The model under review builds one solid part; all positions refer to its coordinate system, in mm. A direction names the side the tool comes from. Give positions to 0.01 mm unless a question says otherwise; leave off trailing zeros. Order: outer loops, then holes, each group sorted by start corner. A loop starts at its lowest first (then second) coordinate and runs counter-clockwise, first axis right, second up. Notation, with made-up numbers: (39, -18) - (73, -18) arc R12 ccw to (73, -6) - close; hole circle Ø6 at (45, 16). An arc over 180 degrees is marked (long way). Use CSV: the item, a comma, the result in double quotes. Start each with the question number.
1. Machinability: for faces 1 (the flat face through (5, 2, -22)), 2 (the flat face through (-22, 2, -5)), 3 (the flat face through (7.42, 3.1, 2.57)), which of the approach directions +Z, -Z, +X, -X, +Y, -Y give a long, thin tool a straight path to every point of the face, cutting with its end or side? Answer none if there is none.
2. To check wall thickness, follow line 1 (Z direction, x = -1, y = 2.9); line 2 (Z direction, x = -27.5, y = 2.85); line 3 (X direction, y = 0.85, z = -22). State the ranges of each line that lie inside material, in increasing order. Write a range as [from, to].
3. Take a section at A-A, the plane x = -24. State the section outline as (y, z) points, then the cut area to 3 significant figures.
4. Draft analysis for pull direction X (two halves, no side actions). For faces 4 (the cylindrical face through (-32.7, 1.7, -0.1)), 5 (the conical face through (-0.817, 0.484, 16.921)), 6 (the flat face through (5, 2, 22)), state which applies: released by +X, released by -X, zero draft, split by the parting line, or undercut.
5. Take a section at B-B, the plane y = 0.85. Count the separate pieces of the cut face and the enclosed holes in it, then the cut area to 3 significant figures.
6. For pin 1 (0.9 mm diameter, centred on x = 22.5, y = 1, fed in from +Z); pin 2 (1.5 mm diameter, centred on x = 12, y = 1, fed in from +Z); pin 3 (0.9 mm diameter, centred on x = 20.5, y = 1.5, fed in from -Z), all flat-tipped, find the tip position at first contact; note any pin that passes through.
```python
from build123d import *

# Parameters (mm, degrees)
SKETCH1_R           = 7.45
SKETCH1_R_2         = 2
BOSS_EXTRUDE1_DEPTH = 3.1
CIRPATTERN1_COUNT   = 4
CHAMFER3_SIZE       = 0.25
CHAMFER4_SIZE       = 2.75
CHAMFER5_SIZE       = 0.25


with BuildPart() as part:
    # Sketch1 → Boss-Extrude1 (new body)
    with BuildSketch(Plane(origin=(0, 0, 0), x_dir=(1, 0, 0), z_dir=(0, 1, 0))):
        with BuildLine():
            Line((5, 16.58427681), (5, 27.7))
            ThreePointArc((5, 27.7), (0, 32.7), (-5, 27.7))
            Line((-5, 27.7), (-5, 16.58427681))
            ThreePointArc((-5, 16.58427681), (-4.969037433, 15.767138405), (-5, 14.95))
            ThreePointArc((-5, 14.95), (-5.95461278, 11.260107735), (-8.131727984, 8.131727984))
            ThreePointArc((-8.131727984, 8.131727984), (0, -11.5), (8.131727984, 8.131727984))
            ThreePointArc((8.131727984, 8.131727984), (5.95461278, 11.260107735), (5, 14.95))
            ThreePointArc((5, 14.95), (4.969037433, 15.767138405), (5, 16.58427681))
        make_face()
        with Locations(Location((0, 0, 0), (0, 0, 90))):
            Circle(SKETCH1_R, mode=Mode.SUBTRACT)
        with Locations(Location((0, 14.95, 0), (0, 0, 90))):
            Circle(SKETCH1_R_2, mode=Mode.SUBTRACT)
        with Locations(Location((0, 27.7, 0), (0, 0, 90))):
            Circle(SKETCH1_R_2, mode=Mode.SUBTRACT)
    extrude(amount=BOSS_EXTRUDE1_DEPTH)


with BuildPart() as cirpattern1_1:
    # CirPattern1: pattern copy
    add(part.part.rotate(Axis((0, 0, 0), (0, 1, 0)), 1 * 360 / CIRPATTERN1_COUNT))


with BuildPart() as cirpattern1_2:
    # CirPattern1: pattern copy
    add(part.part.rotate(Axis((0, 0, 0), (0, 1, 0)), 2 * 360 / CIRPATTERN1_COUNT))


with BuildPart() as cirpattern1_3:
    # CirPattern1: pattern copy
    add(part.part.rotate(Axis((0, 0, 0), (0, 1, 0)), 3 * 360 / CIRPATTERN1_COUNT))


with BuildPart() as cirpattern1_1_1:
    add(cirpattern1_1.part)

    # Combine1: union part, CirPattern1_3, CirPattern1_2
    add(part.part)
    add(cirpattern1_3.part)
    add(cirpattern1_2.part)

    # Chamfer3
    chamfer3_edges = [cirpattern1_1_1.edges().sort_by_distance(p)[0] for p in [
        (-25.7, 3.1, 0),
        (0, 3.1, -25.7),
        (25.7, 3.1, 0),
        (0, 3.1, 25.7),
        (7.45, 3.1, 0),
    ]]
    chamfer(chamfer3_edges, length=CHAMFER3_SIZE)

    # Chamfer4
    chamfer4_edges = [cirpattern1_1_1.edges().sort_by_distance(p)[0] for p in [
        (-12.95, 3.1, 0),
        (0, 3.1, -12.95),
        (12.95, 3.1, 0),
        (0, 3.1, 12.95),
    ]]
    chamfer(chamfer4_edges, length=CHAMFER4_SIZE)

    # Chamfer5
    chamfer5_edges = [cirpattern1_1_1.edges().sort_by_distance(p)[0] for p in [
        (-32.7, 0, 0),
        (-22.142138405, 0, -5),
        (-8.131727984, 0, -8.131727984),
        (-8.131727984, 0, 8.131727984),
        (-22.142138405, 0, 5),
        (-25.7, 0, 0),
        (-12.95, 0, 0),
        (0, 0, -25.7),
        (0, 0, -12.95),
        (8.131727984, 0, -8.131727984),
        (5, 0, -22.142138405),
        (25.7, 0, 0),
        (12.95, 0, 0),
        (8.131727984, 0, 8.131727984),
        (22.142138405, 0, 5),
        (0, 0, 25.7),
        (0, 0, 12.95),
        (-5, 0, 22.142138405),
        (-5, 0, -22.142138405),
        (0, 0, -32.7),
        (22.142138405, 0, -5),
        (32.7, 0, 0),
        (5, 0, 22.142138405),
        (0, 0, 32.7),
    ]]
    chamfer(chamfer5_edges, length=CHAMFER5_SIZE)


solid = cirpattern1_1_1.part
```
Determined:
1,face 1,"-Z, +X, +Y, -Y"
1,face 2,"-Z, -X, +Y, -Y"
1,face 3,"+Z, -Z, +X, -X, +Y"
2,line 1,"z = [-32.6, -29.49], [-25.91, -19.39], [-10.51, -7.43], [7.43, 10.51], [19.39, 25.91], [29.49, 32.6]"
2,line 2,"z = [-5, -1.99], [1.99, 5]"
2,line 3,"x = [-5, 5]"
3,outline,"(0, -4.75) - (0.25, -5) - (3.1, -5) - (3.1, 5) - (0.25, 5) - (0, 4.75) - close"
3,area,"30.9 mm²"
4,face 4,"released by -X"
4,face 5,"undercut"
4,face 6,"released by +X"
5,separate pieces,"1"
5,enclosed holes,"9"
5,area,"959 mm²"
6,pin 1,"stops at z = 5"
6,pin 2,"stops at z = 5.96"
6,pin 3,"stops at z = -5"
